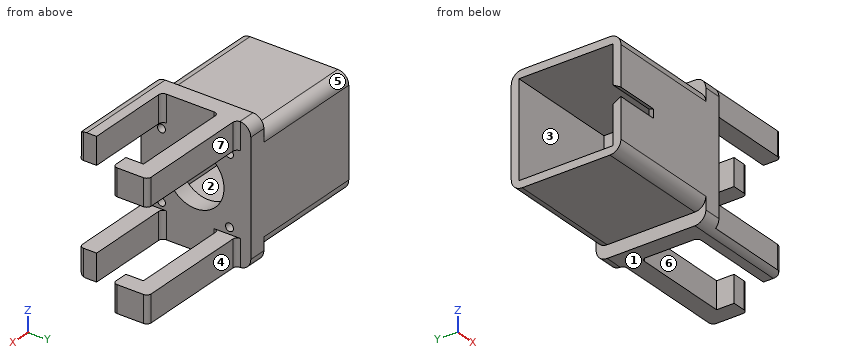
```python
from build123d import *

# Parameters (mm, degrees)
SKETCH1_W                 = 12.25
SKETCH1_H                 = 8
BOSS_EXTRUDE1_DEPTH       = 54
BOSS_EXTRUDE1_2_DEPTH     = 54
SKETCH1_7_W               = 12.25
SKETCH1_7_H               = 8
BOSS_EXTRUDE7_DEPTH       = 40
BOSS_EXTRUDE7_2_DEPTH     = 40
BOSS_EXTRUDE2_START       = -8
BOSS_EXTRUDE2_OUTLINE_W   = 61.55
BOSS_EXTRUDE2_OUTLINE_H   = 50
BOSS_EXTRUDE2_OUTLINE_R   = 1.8
BOSS_EXTRUDE2_OUTLINE_R_2 = 13
BOSS_EXTRUDE2_DEPTH       = 8
FILLET1_R                 = 2
SKETCH2_W                 = 8
SKETCH2_H                 = 12.25
BOSS_EXTRUDE3_DEPTH       = 8
FILLET2_R                 = 5
FILLET3_R                 = 2
SKETCH3_W                 = 50
SKETCH3_H                 = 50
BOSS_EXTRUDE4_DEPTH       = 52
FILLET7_R                 = 5
SKETCH4_W                 = 20
SKETCH4_H                 = 4
CUT_EXTRUDE1_DEPTH        = 3.5
CUT_EXTRUDE1_TAPER        = -30


# Read off the part's stored shape, not the designer's step: Boss-Extrude2
with BuildPart() as part:
    # Sketch1 → Boss-Extrude1 (new body)
    with BuildSketch(Plane(origin=(0, 0, 0), x_dir=(0, 0, -1), z_dir=(1, 0, 0))):
        with Locations((6.125, 39.3)):
            Rectangle(SKETCH1_W, SKETCH1_H)
    extrude(amount=BOSS_EXTRUDE1_DEPTH)



with BuildPart() as body_2:
    # Sketch1 → Boss-Extrude1 2 (new body)
    with BuildSketch(Plane(origin=(0, 0, 0), x_dir=(0, 0, -1), z_dir=(1, 0, 0))):
        with Locations((55.425, 39.3)):
            Rectangle(SKETCH1_W, SKETCH1_H)
    extrude(amount=BOSS_EXTRUDE1_2_DEPTH)


with BuildPart() as body_3:
    # Sketch1<7> → Boss-Extrude7 (new body)
    with BuildSketch(Plane(origin=(0, 0, 0), x_dir=(0, 0, -1), z_dir=(1, 0, 0))):
        with Locations((6.125, 5.5)):
            Rectangle(SKETCH1_7_W, SKETCH1_7_H)
    extrude(amount=BOSS_EXTRUDE7_DEPTH)


with BuildPart() as body_4:
    # Sketch1<7> → Boss-Extrude7 2 (new body)
    with BuildSketch(Plane(origin=(0, 0, 0), x_dir=(0, 0, -1), z_dir=(1, 0, 0))):
        with Locations((55.425, 5.5)):
            Rectangle(SKETCH1_7_W, SKETCH1_7_H)
    extrude(amount=BOSS_EXTRUDE7_2_DEPTH)


with BuildPart() as part_1:
    add(part.part)

    add(body_2.part)  # Boss-Extrude2 merges body 2

    add(body_3.part)  # Boss-Extrude2 merges body 3

    add(body_4.part)  # Boss-Extrude2 merges body 4
    # Boss-Extrude2 outline → Boss-Extrude2 (add)
    with BuildSketch(Plane(origin=(0, 0, 0), x_dir=(0, 0, -1), z_dir=(1, 0, 0)).offset(BOSS_EXTRUDE2_START)):
        with Locations((30.775, 25)):
            Rectangle(BOSS_EXTRUDE2_OUTLINE_W, BOSS_EXTRUDE2_OUTLINE_H)
        with Locations((15.275219356, 9.300219356)):
            Circle(BOSS_EXTRUDE2_OUTLINE_R, mode=Mode.SUBTRACT)
        with Locations((46.274780644, 9.300219356)):
            Circle(BOSS_EXTRUDE2_OUTLINE_R, mode=Mode.SUBTRACT)
        with Locations((30.775, 24.8)):
            Circle(BOSS_EXTRUDE2_OUTLINE_R_2, mode=Mode.SUBTRACT)
        with Locations((15.275219356, 40.299780644)):
            Circle(BOSS_EXTRUDE2_OUTLINE_R, mode=Mode.SUBTRACT)
        with Locations((46.274780644, 40.299780644)):
            Circle(BOSS_EXTRUDE2_OUTLINE_R, mode=Mode.SUBTRACT)
    extrude(amount=BOSS_EXTRUDE2_DEPTH)

    # Fillet1
    fillet1_edges = [part_1.edges().sort_by_distance(p)[0] for p in [
        (0, 35.3, -55.425),
        (0, 43.3, -55.425),
        (0, 35.3, -6.125),
        (0, 9.5, -6.125),
        (0, 43.3, -6.125),
        (0, 9.5, -55.425),
    ]]
    fillet(fillet1_edges, radius=FILLET1_R)

    # Sketch2 → Boss-Extrude3 (add)
    with BuildSketch(Plane.XZ.offset(-35.3)):
        with Locations((50, -6.125)):
            Rectangle(SKETCH2_W, SKETCH2_H)
        with Locations((50, -55.425)):
            Rectangle(SKETCH2_W, SKETCH2_H)
    extrude(amount=BOSS_EXTRUDE3_DEPTH)

    # Fillet2
    fillet2_edges = [part_1.edges().sort_by_distance(p)[0] for p in [
        (-4, 50, -61.55),
        (-4, 0, -61.55),
        (-4, 0, 0),
        (-4, 50, 0),
    ]]
    fillet(fillet2_edges, radius=FILLET2_R)

    # Fillet3
    fillet3_edges = [part_1.edges().sort_by_distance(p)[0] for p in [
        (54, 43.3, -6.125),
        (54, 27.3, -6.125),
        (54, 27.3, -55.425),
        (40, 1.5, -54.710357107),
        (40, 1.5, -6.839642893),
        (54, 43.3, -55.425),
    ]]
    fillet(fillet3_edges, radius=FILLET3_R)

    # Sketch3 → Boss-Extrude4 (add)
    with BuildSketch(Plane.ZY.offset(8)):
        with Locations((-30.775, 25)):
            Rectangle(SKETCH3_W, SKETCH3_H)
        Polygon((-52.275, 46.5), (-9.232535772, 46.5), (-9.275, 3.5), (-52.275, 3.5), align=None, mode=Mode.SUBTRACT)
    extrude(amount=BOSS_EXTRUDE4_DEPTH)

    # Fillet7
    fillet7_edges = [part_1.edges().sort_by_distance(p)[0] for p in [
        (-34, 50, -55.775),
        (-34, 0, -55.775),
        (-34, 0, -5.775),
        (-34, 50, -5.775),
    ]]
    fillet(fillet7_edges, radius=FILLET7_R)

    # Sketch4 → Cut-Extrude1 (cut)
    with BuildSketch(Plane.XZ):
        with Locations((-50, -30.775)):
            Rectangle(SKETCH4_W, SKETCH4_H)
    extrude(amount=-CUT_EXTRUDE1_DEPTH, taper=CUT_EXTRUDE1_TAPER, mode=Mode.SUBTRACT)


solid = part_1.part
```
Here's how the part is built. I have some questions about the finished solid (model axes, mm). Face numbers are marked on the shaded views. A direction names the side the tool comes from. Coordinates: 2 decimals unless noted, no trailing zeros. Loops run counter-clockwise (first coordinate to the right, second up) from the corner with the lowest first, then second, coordinate; pieces in that order, holes last. Notation, with made-up numbers: (3, 18.25) - (26, 18.25) arc R27 ccw to (26, 50.25) - close; hole circle Ø9 at (-35, 1). An arc over 180 degrees is marked (long way). Return JSON: item names as keys, results as strings. Group by question number.
Item 1: We'd pull the mould along Z, two halves only. Please class the marked faces 1, 2, 3 and 4: +Z half, -Z half, draft (parallel to the pull), parting line (faces both ways), or undercut.
Item 2: On a 3-axis mill with a long thin cutter (end or side, diameter ignored), from which of +Z, -Z, +X, -X, +Y, -Y can I reach the whole of each face in a straight line? I mean the marked faces 5, 6 and 7. Say none if no direction works.
Item 3: If we section it at B-B on y = 20.5: Write out the boundary of the cut face in (x, z) (3 decimals), and give its area (3 significant figures).
Item 4: If we section it at C-C on z = -37: Write out the boundary of the cut face in (x, y).
Item 5: Will these pins go through, and if not, where does the flat tip stop? P1, Ø3.5, axis at x = 17, z = -53, coming from the +Y side; P2, Ø5.5, axis at x = 17.5, z = -53, coming from the -Y side; P3, Ø1, axis at x = 1, y = 31, coming from the -Z side; P4, Ø6.5, axis at y = 6.5, z = -56, coming from the +X side.
Item 6: I need wall thicknesses on line 1 (Z direction, x = -13, y = 9.5) (3 decimals); line 2 (Z direction, x = -9.5, y = 32) (3 decimals); line 3 (Y direction, x = -17, z = -12). Which ranges of each line are inside material? Lowest first, please. Write a range as from..to.
Item 7: If we section it at A-A on x = 24: Write out the boundary of the cut face in (y, z).
Item 8: If we section it at D-D on x = -24: Write out the boundary of the cut face in (y, z) (3 decimals), and give its area (3 significant figures).
Calculated:
{
 "1": {"face 1": "-Z half", "face 2": "undercut", "face 3": "undercut", "face 4": "draft"},
 "2": {"face 5": "+Z, -X, +Y", "face 6": "+Z, -Z", "face 7": "+Z, -Z, +X, +Y"},
 "3": {"outline": "(-60, -55.775) - (-8, -55.775) - (-8, -61.55) - (0, -61.55) - (0, -43.043) - (-8, -43.043) - (-8, -52.275) - (-60, -52.275) - close; (-60, -9.258) - (-8, -9.258) - (-8, -18.507) - (0, -18.507) - (0, 0) - (-8, 0) - (-8, -5.775) - (-60, -5.775) - close", "area": "659 mm^2"},
 "4": {"outline": "(-60, 0) - (0, 0) - (0, 13.39) - (-8, 13.39) - (-8, 3.5) - (-60, 3.5) - close; (-60, 46.5) - (-8, 46.5) - (-8, 36.21) - (0, 36.21) - (0, 50) - (-60, 50) - close"},
 "5": {"P1": "stops at y = 43.3", "P2": "stops at y = 1.5", "P3": "passes through", "P4": "stops at x = 40"},
 "6": {"line 1": "z = -55.775..-52.275, -9.269..-5.775", "line 2": "z = -55.775..-52.275, -9.247..-5.775", "line 3": "y = 0..3.5, 46.5..50"},
 "7": {"outline": "(1.5, -60.12) arc R5 ccw to (5, -61.55) - (9.5, -61.55) - (9.5, -49.3) - (1.5, -49.3) - close; (1.5, -12.25) - (9.5, -12.25) - (9.5, 0) - (5, 0) arc R5 ccw to (1.5, -1.43) - close; (35.3, -61.55) - (43.3, -61.55) - (43.3, -49.3) - (35.3, -49.3) - close; (35.3, -12.25) - (43.3, -12.25) - (43.3, 0) - (35.3, 0) - close"},
 "8": {"outline": "(0, -50.775) arc R5 ccw to (5, -55.775) - (45, -55.775) arc R5 ccw to (50, -50.775) - (50, -10.775) arc R5 ccw to (45, -5.775) - (5, -5.775) arc R5 ccw to (0, -10.775) - close; hole (3.5, -52.275) - (46.5, -52.275) - (46.5, -9.233) - (3.5, -9.275) - close", "area": "629 mm^2"}
}
